Model file for the job. Use its own axes, mm. Face numbers are marked on the shaded views. Coordinates: 2 decimals unless noted, no trailing zeros. Write each loop counter-clockwise with the first axis right and the second up, starting at its lowest first coordinate (ties: lowest second). Pieces come first, ordered by that corner, then holes. Notation, with made-up numbers: (71.5, -39.5) -> (114.5, -39.5) arc R32 cw to (114.5, -13.5) -> close; hole circle Ø2 at (-39.5, 28.25). An arc over 180 degrees is marked (long way). Answer as a JSON object with one key per item and string values. Group by question number.
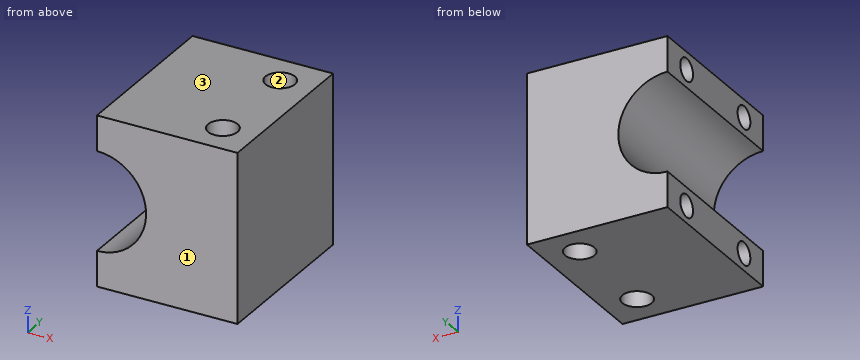
from build123d import *

# Parameters (mm, degrees)
F1_DEPTH = 30
F3_D     = 10.5
F4_D     = 10.5
F6_D     = 8
F6_DEPTH = 20
F6_TIP   = 2.4034424761


with BuildPart() as f1:
    # F0 (on Front) → F1 (new body, symmetric)
    with BuildSketch(Plane.XZ):
        with BuildLine():
            Line((-25, -17.5), (-25, -30))
            Line((-25, -30), (25, -30))
            Line((25, -30), (25, 30))
            Line((25, 30), (-25, 30))
            Line((-25, 30), (-25, 17.5))
            ThreePointArc((-25, 17.5), (-7.5, 0), (-25, -17.5))
        make_face()
    extrude(amount=F1_DEPTH, both=True)

    # F3 (through all)
    with Locations(Plane.XY.offset(30)):
        with Locations((13, 18)):
            Hole(F3_D / 2)

    # F4 (through all)
    with Locations(Plane.XY.offset(30)):
        with Locations((13, -18)):
            Hole(F4_D / 2)

    # F6
    with Locations(Plane(origin=(-25, 0, 0), x_dir=(0, -1, 0), z_dir=(-1, 0, 0))):
        with Locations((18, 23.75), (-18, 23.75), (-18, -24), (18, -24)):
            Hole(F6_D / 2, depth=F6_DEPTH)
            with Locations((0, 0, -(F6_DEPTH + F6_TIP / 2))):  # 118° drill point
                Cone(0, F6_D / 2, F6_TIP, mode=Mode.SUBTRACT)


solid = f1.part
(1) Pull direction Y, two halves, no side cores. Call the marked faces 1, 2 and 3: released by +Y, released by -Y, zero draft, split by the parting line, or undercut.
(2) Cut at A-A on z = 0. List the corners of the cut face in (x, y).
(3) Cut at D-D on z = -12. List the corners of the cut face in (x, y).
(4) Cut at B-B on x = 15. List the corners of the cut face in (y, z).
(5) Pin check, flat tip, straight feed: pin 1 (7 mm diameter, centred on y = 18, z = 23.75, fed in from -X). Stop position of the tip, or through.
(6) Wall check: probe 1 along Y at (x, z) = (13, -11); probe 2 along Y at (x, z) = (-10.5, -24); probe 3 along Z at (x, y) = (-14.5, -18). Give the ranges that are in metal, low to high.
(7) Cut at C-C on y = 0.5. List the corners of the cut face in (x, z), plus the area to 3 significant figures.
Results found:
{
 "1": {"face 1": "released by -Y", "face 2": "undercut", "face 3": "zero draft"},
 "2": {"outline": "(-7.5, -30) -> (25, -30) -> (25, 30) -> (-7.5, 30) -> close; hole circle Ø10.5 at (13, -18); hole circle Ø10.5 at (13, 18)"},
 "3": {"outline": "(-12.26, -30) -> (25, -30) -> (25, 30) -> (-12.26, 30) -> close; hole circle Ø10.5 at (13, -18); hole circle Ø10.5 at (13, 18)"},
 "4": {"outline": "(-30, -30) -> (-22.85, -30) -> (-22.85, 30) -> (-30, 30) -> close; (-13.15, -30) -> (13.15, -30) -> (13.15, 30) -> (-13.15, 30) -> close; (22.85, -30) -> (30, -30) -> (30, 30) -> (22.85, 30) -> close"},
 "5": {"pin 1": "stops at x = -4.7"},
 "6": {"probe 1": "y = -30 to -23.25, -12.75 to 12.75, 23.25 to 30", "probe 2": "y = -30 to -22, -14 to 14, 22 to 30", "probe 3": "z = -30 to -28, -20 to -14, 14 to 19.75, 27.75 to 30"},
 "7": {"outline": "(-25, -30) -> (25, -30) -> (25, 30) -> (-25, 30) -> (-25, 17.5) arc R17.5 cw to (-25, -17.5) -> close", "area": "2,520 mm²"}
}
